For this review, take the finished solid that the model builds, in its own axes (mm). A direction names the side the tool comes from. Give positions to 0.01 mm unless a question says otherwise; leave off trailing zeros. Order: outer loops, then holes, each group sorted by start corner. A loop starts at its lowest first (then second) coordinate and runs counter-clockwise, first axis right, second up. Notation, with made-up numbers: (40, -17.5) - (59, -17.5) arc R15 cw to (59, -10.5) - close; hole circle Ø7 at (35.25, 47). An arc over 180 degrees is marked (long way). Use a Markdown table: item, result. Add a question column.
1) We need section D-D on z = 0. Write out the cut boundary in (x, y).
2) Clearance check with flat-ended pins moving along their axes: P1, Ø10, axis at x = 19.5, z = 16, coming from the -Y side; P2, Ø6.5, axis at x = -25, y = -108, coming from the -Z side; P3, Ø25, axis at x = -15.5, z = 7.5, coming from the +Y side. State where each tip first meets the part, or that it passes through.
3) Machinability: for faces 4 (the face through (26.474, 9.352, 23.479)), 5 (the face through (0, 38, 22)), 6 (the face through (-4, -35, 4)), which of the approach directions +Z, -Z, +X, -X, +Y, -Y give a long, thin tool a straight path to every point of the face, cutting with its end or side? Answer none if there is none.
4) Wall thickness on L1, parallel to Y at x = 25, z = 23.8; L2, parallel to Y at x = -4, z = -4; L3, parallel to Y at x = -17.5, z = 17: over which ranges is each line inside the solid? List them lowest first.
5) We need section A-A on x = -9.5. Write out the cut boundary in (y, z).
6) We need section C-C on y = -71.5. Write out the cut boundary in (x, z).
7) We need section B-B on z = 13.5. Write out the cut boundary in (x, y), then the cut area to 3 significant figures.
8) Mouldability with a two-part tool opening along Y and no side actions: class faces 1 (the face through (0, -136, 25)), 2 (the face through (0, -103, -1)), 3 (the face through (-1.08, -82.26, -4.88)) as released by +Y, released by -Y, zero draft, split by the parting line, or undercut.
```python
from build123d import *

# Parameters (mm, degrees)
SKETCH1_W           = 70
SKETCH1_H           = 50
BOSS_EXTRUDE1_DEPTH = 3
SKETCH2_W           = 70
SKETCH2_H           = 3
BOSS_EXTRUDE2_DEPTH = 70
SKETCH3_R           = 2
CUT_EXTRUDE1_DEPTH  = 6
SKETCH4_R           = 5
BOSS_EXTRUDE3_DEPTH = 35
SKETCH5_R           = 6
BOSS_EXTRUDE4_DEPTH = 30
SKETCH6_R           = 5
BOSS_EXTRUDE5_DEPTH = 35
SKETCH7_W           = 70
SKETCH7_H           = 50
BOSS_EXTRUDE6_DEPTH = 3
SKETCH8_W           = 70
SKETCH8_H           = 3
BOSS_EXTRUDE7_DEPTH = 70
SKETCH9_R           = 2
CUT_EXTRUDE2_DEPTH  = 70


with BuildPart() as part:
    # Sketch1 → Boss-Extrude1 (new body)
    with BuildSketch(Plane(origin=(0, 0, 0), x_dir=(1, 0, 0), z_dir=(0, 1, 0))):
        Rectangle(SKETCH1_W, SKETCH1_H)
    extrude(amount=BOSS_EXTRUDE1_DEPTH)

    # Sketch2 → Boss-Extrude2 (add)
    with BuildSketch(Plane(origin=(0, 3, 0), x_dir=(1, 0, 0), z_dir=(0, 1, 0))):
        with Locations((0, -23.5)):
            Rectangle(SKETCH2_W, SKETCH2_H)
    extrude(amount=BOSS_EXTRUDE2_DEPTH)

    # Sketch3 → Cut-Extrude1 (cut)
    with BuildSketch(Plane(origin=(0, 0, 22), x_dir=(-1, 0, 0), z_dir=(0, 0, -1))):
        with Locations((25, 8)):
            Circle(SKETCH3_R)
        with Locations((-25, 8)):
            Circle(SKETCH3_R)
    extrude(amount=-CUT_EXTRUDE1_DEPTH, mode=Mode.SUBTRACT)

    # Sketch4 → Boss-Extrude3 (add)
    with BuildSketch(Plane.XZ):
        Circle(SKETCH4_R)
    extrude(amount=BOSS_EXTRUDE3_DEPTH)

    # Sketch5 → Boss-Extrude4 (add)
    with BuildSketch(Plane.XZ.offset(35)):
        Circle(SKETCH5_R)
    extrude(amount=BOSS_EXTRUDE4_DEPTH)

    # Sketch6 → Boss-Extrude5 (add)
    with BuildSketch(Plane.XZ.offset(65)):
        Circle(SKETCH6_R)
    extrude(amount=BOSS_EXTRUDE5_DEPTH)

    # Sketch7 → Boss-Extrude6 (add)
    with BuildSketch(Plane.XZ.offset(100)):
        Rectangle(SKETCH7_W, SKETCH7_H)
    extrude(amount=BOSS_EXTRUDE6_DEPTH)

    # Sketch8 → Boss-Extrude7 (add)
    with BuildSketch(Plane.XZ.offset(103)):
        with Locations((0, 23.5)):
            Rectangle(SKETCH8_W, SKETCH8_H)
    extrude(amount=BOSS_EXTRUDE7_DEPTH)

    # Sketch9 → Cut-Extrude2 (cut)
    with BuildSketch(Plane(origin=(0, 0, 22), x_dir=(-1, 0, 0), z_dir=(0, 0, -1))):
        with Locations((-25, -108)):
            Circle(SKETCH9_R)
        with Locations((25, -108)):
            Circle(SKETCH9_R)
    extrude(amount=-CUT_EXTRUDE2_DEPTH, mode=Mode.SUBTRACT)


solid = part.part
```
Checked values:
| question | item | result |
|---|---|---|
| 1 | outline | (-35, -103) - (35, -103) - (35, -100) - (5, -100) - (5, -65) - (6, -65) - (6, -35) - (5, -35) - (5, 0) - (35, 0) - (35, 3) - (-35, 3) - (-35, 0) - (-5, 0) - (-5, -35) - (-6, -35) - (-6, -65) - (-5, -65) - (-5, -100) - (-35, -100) - close |
| 2 | P1 | y = -103 |
| 2 | P2 | z = 22 |
| 2 | P3 | y = 3 |
| 3 | face 4 | +Z, -Z |
| 3 | face 5 | -Z, +X, -X, +Y |
| 3 | face 6 | none |
| 4 | L1 | -173 to -110, -106 to -100, 0 to 6, 10 to 73 |
| 4 | L2 | -103 to -100, -65 to -35, 0 to 3 |
| 4 | L3 | -103 to -100, 0 to 3 |
| 5 | outline | (-173, 22) - (-103, 22) - (-103, -25) - (-100, -25) - (-100, 25) - (-173, 25) - close; (0, -25) - (3, -25) - (3, 22) - (73, 22) - (73, 25) - (0, 25) - close |
| 6 | outline | circle Ø10 at (0, 0) |
| 7 | outline | (-35, -103) - (35, -103) - (35, -100) - (-35, -100) - close; (-35, 0) - (35, 0) - (35, 3) - (-35, 3) - close |
| 7 | area | 420 mm² |
| 8 | face 1 | zero draft |
| 8 | face 2 | released by -Y |
| 8 | face 3 | undercut |
